Could you check a few things on this model? Use its own coordinates, in mm. Round coordinates to 2 decimals unless told otherwise and drop trailing zeros. Write each loop counter-clockwise with the first axis right and the second up, starting at its lowest first coordinate (ties: lowest second). Pieces come first, ordered by that corner, then holes. Notation, with made-up numbers: (59.25, 64) -> (118.25, 64) arc R31 ccw to (118.25, 96) -> close; hole circle Ø9 at (64.25, 70.25). An arc over 180 degrees is marked (long way). One line per question, with ' | ' between items. Start each with the question number.
1. If I drill on line 1 along Z through (x, y) = (-2.5, -1.15); line 2 along X through (y, z) = (-0.1, 1.5); line 3 along Y through (x, z) = (-1, 9.75), over which ranges is the centre line in solid material (lowest first)? Write a range as [from, to].
2. Imagine slicing it at A-A, the plane z = 14.5. List the corners of the cut face in (x, y) for me.
3. Imagine slicing it at D-D, the plane y = -0.85. List the corners of the cut face in (x, z) for me.
4. For pin 1 Ø2 at (x, y) = (2, 1.5) entering from +Z; pin 2 Ø1 at (x, z) = (-0.5, 0) entering from +Y; pin 3 Ø3 at (x, z) = (1, 10) entering from -Y, each with a flat end and sliding along its axis, tell me the tip position at first contact or that it passes through.
5. Imagine slicing it at C-C, the plane x = 0. List the corners of the cut face in (y, z) for me, and give its area (3 significant figures).
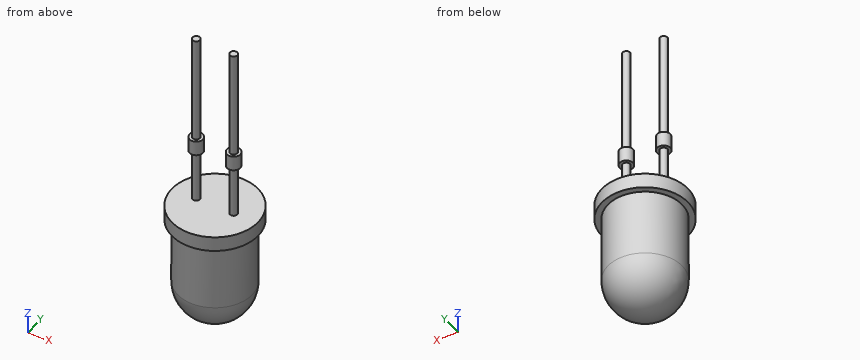
from build123d import *

# Parameters (mm, degrees)
SKETCH_1_R          = 2.5
EXTRUDE_1_DEPTH     = 5.5
SKETCH_2_R          = 2.9
EXTRUDE_2_DEPTH     = 1
SKETCH_3_R          = 0.25
EXTRUDE_3_DEPTH     = 12.7
SKETCH_6_R          = 0.45
SKETCH_6_R_2        = 0.25
EXTRUDE_1_2_DEPTH   = 4.5
SKETCH_7_R          = 0.45
SKETCH_7_R_2        = 0.25
CUT_EXTRUDE_2_DEPTH = 3.5


with BuildPart() as part:
    # 草图1 → Extrude 1 (new body)
    with BuildSketch(Plane.XY):
        Circle(SKETCH_1_R)
    extrude(amount=EXTRUDE_1_DEPTH)

    # 草图2 → 拉伸2 (add)
    with BuildSketch(Plane.XY.offset(5.5)):
        Circle(SKETCH_2_R)
    extrude(amount=-EXTRUDE_2_DEPTH)

    # 草图3 → 拉伸3 (add)
    with BuildSketch(Plane(origin=(0, 0, 4.5), x_dir=(-1, 0, 0), z_dir=(0, 0, -1))):
        with Locations((-1.27, 0)):
            Circle(SKETCH_3_R)
        with Locations(Location((1.27, 0, 0), (0, 0, 180))):
            Circle(SKETCH_3_R)
    extrude(amount=-EXTRUDE_3_DEPTH)

    # 草图5 → 旋转2 (revolve)
    with BuildSketch(Plane(origin=(0, 0, 0), x_dir=(0, 0, -1), z_dir=(1, 0, 0)), mode=Mode.PRIVATE) as revolve_2_sk:
        with BuildLine():
            Line((0, 2.5), (0, 0))
            Line((0, 0), (2.5, 0))
            ThreePointArc((2.5, 0), (1.767766953, 1.767766953), (0, 2.5))
        make_face()
    revolve(revolve_2_sk.sketch.rotate(Axis((0, 0, -2.5), (0, 0, 1)), 90), axis=Axis((0, 0, -2.5), (0, 0, 1)))

    # 草图6 → Extrude 1 2 (add)
    # profile 1 of 2: a face of its own
    with BuildSketch(Plane.XY.offset(5.5)):
        with Locations((-1.27, 0)):
            Circle(SKETCH_6_R)
        with Locations((-1.27, 0)):
            Circle(SKETCH_6_R_2, mode=Mode.SUBTRACT)
    # profile 2 of 2: a face of its own
    with BuildSketch(Plane.XY.offset(5.5)):
        with Locations((1.27, 0)):
            Circle(SKETCH_6_R)
        with Locations(Location((1.27, 0, 0), (0, 0, 180))):
            Circle(SKETCH_6_R_2, mode=Mode.SUBTRACT)
    extrude(amount=EXTRUDE_1_2_DEPTH)

    # 草图7 → 切除-拉伸2 (cut)
    # profile 1 of 2: a face of its own
    with BuildSketch(Plane.XY.offset(5.5)):
        with Locations((-1.27, 0)):
            Circle(SKETCH_7_R)
        with Locations((-1.27, 0)):
            Circle(SKETCH_7_R_2, mode=Mode.SUBTRACT)
    # profile 2 of 2: a face of its own
    with BuildSketch(Plane.XY.offset(5.5)):
        with Locations((1.27, 0)):
            Circle(SKETCH_7_R)
        with Locations((1.27, 0)):
            Circle(SKETCH_7_R_2, mode=Mode.SUBTRACT)
    extrude(amount=CUT_EXTRUDE_2_DEPTH, mode=Mode.SUBTRACT)


solid = part.part
Geometry results:
1) line 1: z = [4.5, 5.5] | line 2: x = [-2.5, 2.5] | line 3: y = [-0.36, 0.36]
2) outline: circle Ø0.5 at (-1.27, 0); circle Ø0.5 at (1.27, 0)
3) outline: (-2.77, 4.5) -> (-2.35, 4.5) -> (-2.35, 0) arc R2.35 ccw to (2.35, 0) -> (2.35, 4.5) -> (2.77, 4.5) -> (2.77, 5.5) -> (-2.77, 5.5) -> close
4) pin 1: stops at z = 5.5 | pin 2: stops at y = 2.5 | pin 3: stops at y = -0.45
5) outline: (-2.9, 4.5) -> (-2.5, 4.5) -> (-2.5, 0) arc R2.5 ccw to (2.5, 0) -> (2.5, 4.5) -> (2.9, 4.5) -> (2.9, 5.5) -> (-2.9, 5.5) -> close | area: 38.1 mm2
